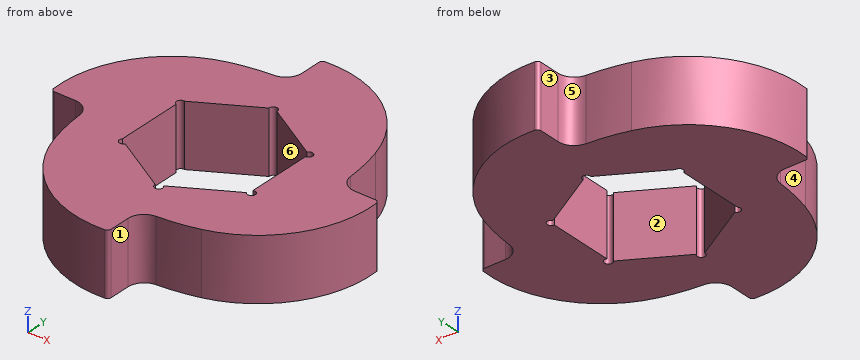
```python
from build123d import *

# Parameters (mm, degrees)
SKETCH1_R           = 16
BOSS_EXTRUDE1_DEPTH = 6.35
SKETCH2_OUTSIDE_W   = 43.14
SKETCH2_OUTSIDE_H   = 43.14
CUT_EXTRUDE1_DEPTH  = 7.35
CUT_EXTRUDE2_DEPTH  = 7.35
CUT_EXTRUDE3_REACH  = 8.35
SKETCH4_R           = 0.4


with BuildPart() as part:
    # Sketch1 → Boss-Extrude1 (new body)
    with BuildSketch(Plane.XY):
        Circle(SKETCH1_R)
    extrude(amount=BOSS_EXTRUDE1_DEPTH)

    # Sketch2 outside → Cut-Extrude1 (cut, through all)
    with BuildSketch(Plane.XY.offset(6.35)):
        Rectangle(SKETCH2_OUTSIDE_W, SKETCH2_OUTSIDE_H)
        with BuildLine():
            Line((14.949348906, 1.700814958), (12.823807348, 1.700814958))
            ThreePointArc((12.823807348, 1.700814958), (11.700778028, 2.141605825), (11.177410812, 3.228610057))
            ThreePointArc((11.177410812, 3.228610057), (10.921226769, 5.268595293), (10.461728017, 7.272599017))
            ThreePointArc((10.461728017, 7.272599017), (6.02807025, 13.518558738), (-1.353723941, 15.562684117))
            ThreePointArc((-1.353723941, 15.562684117), (-1.605363135, 15.44226057), (-1.707494519, 15.182658383))
            Line((-1.707494519, 15.182658383), (-1.707494519, 13.057116825))
            ThreePointArc((-1.707494519, 13.057116825), (-2.148285386, 11.934087504), (-3.235289619, 11.410720289))
            ThreePointArc((-3.235289619, 11.410720289), (-5.275274855, 11.154536246), (-7.279278578, 10.695037493))
            ThreePointArc((-7.279278578, 10.695037493), (-13.525238299, 6.261379727), (-15.569363679, -1.120414464))
            ThreePointArc((-15.569363679, -1.120414464), (-15.448940131, -1.372053658), (-15.189337945, -1.474185042))
            Line((-15.189337945, -1.474185042), (-13.063796386, -1.474185042))
            ThreePointArc((-13.063796386, -1.474185042), (-11.940767066, -1.914975909), (-11.417399851, -3.001980142))
            ThreePointArc((-11.417399851, -3.001980142), (-11.161215808, -5.041965378), (-10.701717055, -7.045969101))
            ThreePointArc((-10.701717055, -7.045969101), (-6.268059288, -13.291928823), (1.113734902, -15.336054202))
            ThreePointArc((1.113734902, -15.336054202), (1.365374097, -15.215630654), (1.467505481, -14.956028468))
            Line((1.467505481, -14.956028468), (1.467505481, -12.830486909))
            ThreePointArc((1.467505481, -12.830486909), (1.908296348, -11.707457589), (2.99530058, -11.184090374))
            ThreePointArc((2.99530058, -11.184090374), (5.035285816, -10.927906331), (7.03928954, -10.468407578))
            ThreePointArc((7.03928954, -10.468407578), (13.285249261, -6.034749811), (15.32937464, 1.347044379))
            ThreePointArc((15.32937464, 1.347044379), (15.208951093, 1.598683573), (14.949348906, 1.700814958))
        make_face(mode=Mode.SUBTRACT)
    extrude(amount=-CUT_EXTRUDE1_DEPTH, mode=Mode.SUBTRACT)

    # Sketch3 → Cut-Extrude2 (cut, through all)
    with BuildSketch(Plane.XY.offset(6.35)):
        Polygon((0, 7.505553499), (-6.5, 3.75277675), (-6.5, -3.75277675), (0, -7.505553499), (6.5, -3.75277675), (6.5, 3.75277675), align=None)
    extrude(amount=-CUT_EXTRUDE2_DEPTH, mode=Mode.SUBTRACT)

    # Sketch4 → Cut-Extrude3 (cut, up to next)
    with BuildSketch(Plane(origin=(0, 0, 0), x_dir=(-1, 0, 0), z_dir=(0, 0, -1)), mode=Mode.PRIVATE) as cut_extrude3_sk1:
        with Locations((-6.5, 3.75277675)):
            Circle(SKETCH4_R)
    cut_extrude3_tool1 = extrude(cut_extrude3_sk1.sketch, amount=-CUT_EXTRUDE3_REACH, mode=Mode.PRIVATE) & part.part
    add(cut_extrude3_tool1.solids().sort_by_distance((6.5, 3.752777, 0))[0], mode=Mode.SUBTRACT)
    # Sketch4 → Cut-Extrude3 (cut, up to next)
    with BuildSketch(Plane(origin=(0, 0, 0), x_dir=(-1, 0, 0), z_dir=(0, 0, -1)), mode=Mode.PRIVATE) as cut_extrude3_sk2:
        with Locations((0, 7.332348419)):
            Circle(SKETCH4_R)
    cut_extrude3_tool2 = extrude(cut_extrude3_sk2.sketch, amount=-CUT_EXTRUDE3_REACH, mode=Mode.PRIVATE) & part.part
    add(cut_extrude3_tool2.solids().sort_by_distance((0, 7.332348, 0))[0], mode=Mode.SUBTRACT)
    # Sketch4 → Cut-Extrude3 (cut, up to next)
    with BuildSketch(Plane(origin=(0, 0, 0), x_dir=(-1, 0, 0), z_dir=(0, 0, -1)), mode=Mode.PRIVATE) as cut_extrude3_sk3:
        with Locations((6.35, 3.492969129)):
            Circle(SKETCH4_R)
    cut_extrude3_tool3 = extrude(cut_extrude3_sk3.sketch, amount=-CUT_EXTRUDE3_REACH, mode=Mode.PRIVATE) & part.part
    add(cut_extrude3_tool3.solids().sort_by_distance((-6.35, 3.492969, 0))[0], mode=Mode.SUBTRACT)
    # Sketch4 → Cut-Extrude3 (cut, up to next)
    with BuildSketch(Plane(origin=(0, 0, 0), x_dir=(-1, 0, 0), z_dir=(0, 0, -1)), mode=Mode.PRIVATE) as cut_extrude3_sk4:
        with Locations((6.2, -3.92598183)):
            Circle(SKETCH4_R)
    cut_extrude3_tool4 = extrude(cut_extrude3_sk4.sketch, amount=-CUT_EXTRUDE3_REACH, mode=Mode.PRIVATE) & part.part
    add(cut_extrude3_tool4.solids().sort_by_distance((-6.2, -3.925982, 0))[0], mode=Mode.SUBTRACT)
    # Sketch4 → Cut-Extrude3 (cut, up to next)
    with BuildSketch(Plane(origin=(0, 0, 0), x_dir=(-1, 0, 0), z_dir=(0, 0, -1)), mode=Mode.PRIVATE) as cut_extrude3_sk5:
        with Locations((-0.3, -7.505553499)):
            Circle(SKETCH4_R)
    cut_extrude3_tool5 = extrude(cut_extrude3_sk5.sketch, amount=-CUT_EXTRUDE3_REACH, mode=Mode.PRIVATE) & part.part
    add(cut_extrude3_tool5.solids().sort_by_distance((0.3, -7.505553, 0))[0], mode=Mode.SUBTRACT)
    # Sketch4 → Cut-Extrude3 (cut, up to next)
    with BuildSketch(Plane(origin=(0, 0, 0), x_dir=(-1, 0, 0), z_dir=(0, 0, -1)), mode=Mode.PRIVATE) as cut_extrude3_sk6:
        with Locations((-6.65, -3.666174209)):
            Circle(SKETCH4_R)
    cut_extrude3_tool6 = extrude(cut_extrude3_sk6.sketch, amount=-CUT_EXTRUDE3_REACH, mode=Mode.PRIVATE) & part.part
    add(cut_extrude3_tool6.solids().sort_by_distance((6.65, -3.666174, 0))[0], mode=Mode.SUBTRACT)


solid = part.part
```
Work out the finished part from the listing and answer in its coordinate system (mm). Face numbers are marked on the shaded views. A direction names the side the tool comes from. Coordinates: 2 decimals unless noted, no trailing zeros. Loops run counter-clockwise (first coordinate to the right, second up) from the corner with the lowest first, then second, coordinate; pieces in that order, holes last. Notation, with made-up numbers: M 77.5,54 L 129.5,54 A30 cw 129.5,85 Z; hole C 60.5,31 d9. An arc over 180 degrees is marked long. Use CSV: the item, a comma, the result in double quotes. Start each with the question number.
(1) Consider line 1 (Y direction, x = 5.5, z = 5.75); line 2 (X direction, y = -3, z = 1.5); line 3 (Y direction, x = -6.2, z = 2.75). Determine where each line is inside the solid, lowest interval first.
(2) Find section C-C, the plane y = -0.5. Give the vertices of the cut face in (x, z), then the cut area to 3 significant figures.
(3) Find section B-B, the plane x = 2. Give the vertices of the cut face in (y, z), then the cut area to 3 significant figures.
(4) For the marked faces 1, 2 and 3, determine the directions among +Z, -Z, +X, -X, +Y, -Y from which every point of the face is accessible in a straight line to the end or side of a thin tool.
(5) Find section D-D, the plane y = -10. Give the vertices of the cut face in (x, z).
(6) For a pull along Y with two mould halves and no side action, classify the marked faces 4, 5 and 6 as +Y half, -Y half, draft (parallel to the pull), parting line (faces both ways), or undercut.
(7) Given pin 1 Ø1.7 at (x, z) = (-13.5, 4) entering from -Y; pin 2 Ø3 at (x, z) = (-11.5, 2) entering from -Y; pin 3 Ø1.7 at (y, z) = (14, 4) entering from -X, each flat-ended and moving along its own axis, determine where each tip first touches the part or whether it passes through.
Recorded:
1,line 1,"y = -10.84 to -4.33, 4.33 to 13.87"
1,line 2,"x = -11.42 to -6.5, 6.5 to 14.8"
1,line 3,"y = -13.34 to -4.33, 3.93 to 10.97"
2,outline,"M -15.6,0 L -6.5,0 L -6.5,6.35 L -15.6,6.35 Z; M 6.5,0 L 15.31,0 L 15.31,6.35 L 6.5,6.35 Z"
2,area,"114 mm^2"
3,outline,"M -11.62,0 L -6.35,0 L -6.35,6.35 L -11.62,6.35 Z; M 6.35,0 L 15.31,0 L 15.31,6.35 L 6.35,6.35 Z"
3,area,"90.3 mm^2"
4,face 1,"+Z, -Z, +X, -Y"
4,face 2,"+Z, -Z"
4,face 3,"+Z, -Z, -X, +Y"
5,outline,"M -9.39,0 L 8.37,0 L 8.37,6.35 L -9.39,6.35 Z"
6,face 4,"-Y half"
6,face 5,"+Y half"
6,face 6,"undercut"
7,pin 1,"stops at y = -1.53"
7,pin 2,"stops at y = -8.9"
7,pin 3,"stops at x = -1.71"
